Part model, mm, in its own coordinate system. Face numbers are marked on the shaded views. A direction names the side the tool comes from. Coordinates: 2 decimals unless noted, no trailing zeros. Loops run counter-clockwise (first coordinate to the right, second up) from the corner with the lowest first, then second, coordinate; pieces in that order, holes last.
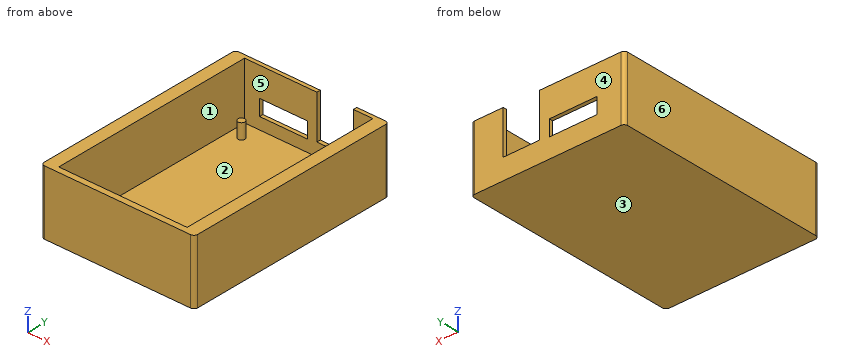
```python
from build123d import *

# Parameters (mm, degrees)
SKETCH_W          = 32.3725
SKETCH_H          = 52.06
SKETCH_R          = 0.6
SKETCH_R_2        = 0.51
SKETCH_R_3        = 1.27
SKETCH_R_4        = 0.45
SKETCH_R_5        = 0.4
SKETCH_R_6        = 0.85
SKETCH_R_7        = 1
SKETCH_R_8        = 0.65
SKETCH_R_9        = 0.405
SKETCH_R_10       = 0.55
SKETCH_R_11       = 0.5
PAD_DEPTH         = 0.1
SKETCH002_W       = 40.3725
SKETCH002_H       = 56.06
PAD001_DEPTH      = 10.9
PAD001_DEPTH_BACK = 6
SKETCH003_W       = 33.7725
SKETCH003_H       = 14.9
POCKET_DEPTH      = 54.5
SKETCH004_R       = 0.9
PAD002_DEPTH      = 4
SKETCH005_W       = 40.3725
SKETCH005_H       = 16.9
PAD003_DEPTH      = 1
SKETCH006_W       = 12.565357
SKETCH006_H       = 4.17396
SKETCH006_W_2     = 9.608805
SKETCH006_H_2     = 11.565347
POCKET001_DEPTH   = 5
FILLET_R          = 1
FILLET001_R       = 1
FILLET002_R       = 0.9
FILLET003_R       = 0.9


with BuildPart() as part:
    # Sketch → Pad (new body)
    with BuildSketch(Plane.XY):
        with Locations((16.18625, 26.03)):
            Rectangle(SKETCH_W, SKETCH_H)
        with Locations((8.1, 2.23)):
            Circle(SKETCH_R, mode=Mode.SUBTRACT)
        with Locations((8.26, 43.82)):
            Circle(SKETCH_R_2, mode=Mode.SUBTRACT)
        with Locations((13.97, 2.54)):
            Circle(SKETCH_R_3, mode=Mode.SUBTRACT)
        with Locations((17.78, 35.56)):
            Circle(SKETCH_R_4, mode=Mode.SUBTRACT)
        with Locations((16.19, 22.23)):
            Circle(SKETCH_R_5, mode=Mode.SUBTRACT)
        with Locations((16.19, 24.77)):
            Circle(SKETCH_R_5, mode=Mode.SUBTRACT)
        with Locations((13.65, 22.23)):
            Circle(SKETCH_R_5, mode=Mode.SUBTRACT)
        with Locations((13.65, 24.77)):
            Circle(SKETCH_R_5, mode=Mode.SUBTRACT)
        with Locations((15.24, 35.56)):
            Circle(SKETCH_R_4, mode=Mode.SUBTRACT)
        with Locations((10.55, 31.43)):
            Circle(SKETCH_R_6, mode=Mode.SUBTRACT)
        with Locations((10.55, 6.03)):
            Circle(SKETCH_R_6, mode=Mode.SUBTRACT)
        with Locations((17.36, 11.6275)):
            Circle(SKETCH_R_7, mode=Mode.SUBTRACT)
        with Locations((13.65, 19.69)):
            Circle(SKETCH_R_5, mode=Mode.SUBTRACT)
        with Locations((16.19, 19.69)):
            Circle(SKETCH_R_5, mode=Mode.SUBTRACT)
        with Locations((13.34, 43.82)):
            Circle(SKETCH_R_2, mode=Mode.SUBTRACT)
        with Locations((10.79, 43.82)):
            Circle(SKETCH_R_2, mode=Mode.SUBTRACT)
        with Locations((18.41, 41.91)):
            Circle(SKETCH_R_8, mode=Mode.SUBTRACT)
        with Locations((30.1625, 2.54)):
            Circle(SKETCH_R_3, mode=Mode.SUBTRACT)
        with Locations((28.36, 11.6275)):
            Circle(SKETCH_R_7, mode=Mode.SUBTRACT)
        with Locations((29.21, 29.53)):
            Circle(SKETCH_R_9, mode=Mode.SUBTRACT)
        with Locations((29.21, 24.45)):
            Circle(SKETCH_R_9, mode=Mode.SUBTRACT)
        with Locations((29.21, 16.83)):
            Circle(SKETCH_R_9, mode=Mode.SUBTRACT)
        with Locations((25.36, 23.54)):
            Circle(SKETCH_R_10, mode=Mode.SUBTRACT)
        with Locations((25.36, 1.63)):
            Circle(SKETCH_R_11, mode=Mode.SUBTRACT)
        with Locations((25.36, 4.13)):
            Circle(SKETCH_R_11, mode=Mode.SUBTRACT)
        with Locations((25.36, 28.54)):
            Circle(SKETCH_R_10, mode=Mode.SUBTRACT)
        with Locations((22.86, 1.63)):
            Circle(SKETCH_R_11, mode=Mode.SUBTRACT)
        with Locations((22.86, 4.13)):
            Circle(SKETCH_R_11, mode=Mode.SUBTRACT)
        with Locations((20.36, 1.63)):
            Circle(SKETCH_R_11, mode=Mode.SUBTRACT)
        with Locations((20.36, 4.13)):
            Circle(SKETCH_R_11, mode=Mode.SUBTRACT)
        with Locations((20.32, 35.56)):
            Circle(SKETCH_R_4, mode=Mode.SUBTRACT)
        with Locations((20.36, 23.54)):
            Circle(SKETCH_R_10, mode=Mode.SUBTRACT)
        with Locations((20.36, 28.54)):
            Circle(SKETCH_R_10, mode=Mode.SUBTRACT)
        with Locations((23.12, 44.91)):
            Circle(SKETCH_R_8, mode=Mode.SUBTRACT)
        with Locations((23.12, 38.91)):
            Circle(SKETCH_R_8, mode=Mode.SUBTRACT)
        with Locations((29.21, 37.15)):
            Circle(SKETCH_R_9, mode=Mode.SUBTRACT)
        with Locations((30.1625, 49.53)):
            Circle(SKETCH_R_3, mode=Mode.SUBTRACT)
        with Locations((4.6, 35.23)):
            Circle(SKETCH_R, mode=Mode.SUBTRACT)
        with Locations((4.6, 2.23)):
            Circle(SKETCH_R, mode=Mode.SUBTRACT)
        with Locations((5.71, 43.82)):
            Circle(SKETCH_R_2, mode=Mode.SUBTRACT)
        with Locations((2.15, 7.33)):
            Circle(SKETCH_R_6, mode=Mode.SUBTRACT)
        with Locations((2.54, 49.53)):
            Circle(SKETCH_R_3, mode=Mode.SUBTRACT)
        with Locations((2.15, 30.13)):
            Circle(SKETCH_R_6, mode=Mode.SUBTRACT)
    extrude(amount=PAD_DEPTH)

    # Sketch002 → Pad001 (new body, two sides)
    with BuildSketch(Plane.XY.offset(0.1)) as pad001_sk:
        with Locations((16.18625, 26.03)):
            Rectangle(SKETCH002_W, SKETCH002_H)
    extrude(amount=PAD001_DEPTH)
    extrude(pad001_sk.sketch, amount=-PAD001_DEPTH_BACK)

    # Sketch003 → Pocket (cut)
    with BuildSketch(Plane(origin=(0, 54.06, 0), x_dir=(-1, 0, 0), z_dir=(0, 1, 0))):
        with Locations((-16.18625, 3.55)):
            Rectangle(SKETCH003_W, SKETCH003_H)
    extrude(amount=-POCKET_DEPTH, mode=Mode.SUBTRACT)

    # Sketch004 → Pad002 (new body)
    with BuildSketch(Plane.XY.offset(-3.9)):
        with Locations((2.533148, 49.528465)):
            Circle(SKETCH004_R)
        with Locations((30.161428, 49.528465)):
            Circle(SKETCH004_R)
        with Locations((30.161428, 2.570097)):
            Circle(SKETCH004_R)
        with Locations((13.958012, 2.570097)):
            Circle(SKETCH004_R)
    extrude(amount=PAD002_DEPTH)

    # Sketch005 → Pad003 (new body)
    with BuildSketch(Plane(origin=(0, 54.06, 0), x_dir=(-1, 0, 0), z_dir=(0, 1, 0))):
        with Locations((-16.18625, 2.55)):
            Rectangle(SKETCH005_W, SKETCH005_H)
    extrude(amount=PAD003_DEPTH)

    # Sketch006 → Pocket001 (cut)
    with BuildSketch(Plane(origin=(0, 55.06, 0), x_dir=(-1, 0, 0), z_dir=(0, 1, 0))):
        with Locations((-9.507967, 1.278049)):
            Rectangle(SKETCH006_W, SKETCH006_H)
        with Locations((-23.116813, 5.321573)):
            Rectangle(SKETCH006_W_2, SKETCH006_H_2)
    extrude(amount=-POCKET001_DEPTH, mode=Mode.SUBTRACT)

    # Fillet
    fillet_edges = [part.edges().sort_by_distance(p)[0] for p in [
        (36.3725, -2, 2.55),
    ]]
    fillet(fillet_edges, radius=FILLET_R)

    # Fillet001
    fillet001_edges = [part.edges().sort_by_distance(p)[0] for p in [
        (-4, -2, 2.55),
    ]]
    fillet(fillet001_edges, radius=FILLET001_R)

    # Fillet002
    fillet002_edges = [part.edges().sort_by_distance(p)[0] for p in [
        (36.3725, 55.06, 2.55),
    ]]
    fillet(fillet002_edges, radius=FILLET002_R)

    # Fillet003
    fillet003_edges = [part.edges().sort_by_distance(p)[0] for p in [
        (-4, 55.06, 2.55),
    ]]
    fillet(fillet003_edges, radius=FILLET003_R)


solid = part.part
```
Q1. Drop flat-ended pins along their axis: P1, Ø1.1, axis at y = 54.5, z = 1, coming from the +X side; P2, Ø6, axis at x = 27, y = 18.5, coming from the +Z side; P3, Ø1.1, axis at x = 25, y = 54.5, coming from the +Z side; P4, Ø0.5, axis at y = 54.5, z = 0.5, coming from the -X side. Give the stop position or say it passes through.
Q2. Saw through at C-C (y = 37). List the corners of the cut face in (x, z), plus the area to 3 significant figures.
Q3. Saw through at A-A (x = 14). List the corners of the cut face in (y, z), plus the area to 3 significant figures.
Q4. Tool access for the marked faces 5 and 6: list every direction of +Z, -Z, +X, -X, +Y, -Y with a clear straight run to the whole face (end or side of a thin tool).
Q5. Saw through at B-B (z = 4.5). List the corners of the cut face in (x, y), plus the area to 3 significant figures.
Q6. Saw through at D-D (z = -2.5). List the corners of the cut face in (x, y), plus the area to 3 significant figures.
Q7. Probe line 1 (Y direction, x = 7, z = 5); line 2 (X direction, y = 40, z = 6); line 3 (Y direction, x = 3, z = -2.5). List the from-to ranges inside material, lowest first.
Q8. Mould opens along Y. For the marked faces 1, 2, 3 and 4 say: released by +Y, released by -Y, zero draft, split by the parting line, or undercut.
Checked values:
1. P1: stops at x = 36.37
1. P2: stops at z = -3.9
1. P3: stops at z = -0.46
1. P4: stops at x = -4
2. outline: (-4, -5.9) - (36.37, -5.9) - (36.37, 11) - (33.07, 11) - (33.07, -3.9) - (-0.7, -3.9) - (-0.7, 11) - (-4, 11) - close
2. area: 179 mm2
3. outline: (-2, -5.9) - (55.06, -5.9) - (55.06, -0.81) - (54.06, -0.81) - (54.06, -3.9) - (3.47, -3.9) - (3.47, 0.1) - (1.67, 0.1) - (1.67, -3.9) - (-0.44, -3.9) - (-0.44, 11) - (-2, 11) - close; (54.06, 3.37) - (55.06, 3.37) - (55.06, 11) - (54.06, 11) - close
3. area: 155 mm2
4. face 5: +Z
4. face 6: +Z, -Z, -X, +Y, -Y
5. outline: (-4, -1) arc R1 ccw to (-3, -2) - (35.37, -2) arc R1 ccw to (36.37, -1) - (36.37, 54.16) arc R0.9 ccw to (35.47, 55.06) - (27.92, 55.06) - (27.92, 54.06) - (33.07, 54.06) - (33.07, -0.44) - (-0.7, -0.44) - (-0.7, 54.06) - (18.31, 54.06) - (18.31, 55.06) - (-3.1, 55.06) arc R0.9 ccw to (-4, 54.16) - close
5. area: 453 mm2
6. outline: (-4, -1) arc R1 ccw to (-3, -2) - (35.37, -2) arc R1 ccw to (36.37, -1) - (36.37, 54.16) arc R0.9 ccw to (35.47, 55.06) - (-3.1, 55.06) arc R0.9 ccw to (-4, 54.16) - close; circle Ø1.8 at (2.53, 49.53); circle Ø1.8 at (13.96, 2.57); circle Ø1.8 at (30.16, 2.57); circle Ø1.8 at (30.16, 49.53); hole (-0.7, -0.44) - (33.07, -0.44) - (33.07, 54.06) - (-0.7, 54.06) - close
6. area: 472 mm2
7. line 1: y = -2 to -0.44, 54.06 to 55.06
7. line 2: x = -4 to -0.7, 33.07 to 36.37
7. line 3: y = -2 to -0.44, 48.76 to 50.3, 54.06 to 55.06
8. face 1: undercut
8. face 2: undercut
8. face 3: zero draft
8. face 4: released by +Y
